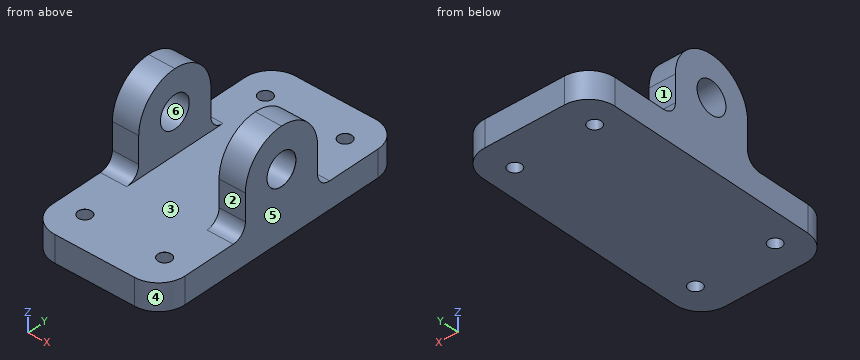
```python
from build123d import *

# Parameters (mm, degrees)
SKETCH1_W                        = 100
SKETCH1_H                        = 50
BOSS_EXTRUDE1_DEPTH              = 10
SKETCH2_W                        = 30
SKETCH2_H                        = 9.9
BOSS_EXTRUDE2_DEPTH              = 30
FILLET1_R                        = 15
F_12_0MM_DOWEL_HOLE1_D           = 12
F_12_0MM_DOWEL_HOLE1_CSINK_D     = 12.05
F_12_0MM_DOWEL_HOLE1_CSINK_ANGLE = 90
F_5_0MM_DOWEL_HOLE1_D            = 5
F_5_0MM_DOWEL_HOLE1_CSINK_D      = 5.05
F_5_0MM_DOWEL_HOLE1_CSINK_ANGLE  = 90
FILLET2_R                        = 5
FILLET3_R                        = 10


with BuildPart() as part:
    # Sketch1 → Boss-Extrude1 (new body)
    with BuildSketch(Plane(origin=(0, 0, 0), x_dir=(0, 1, 0), z_dir=(0, 0, 1))):
        Rectangle(SKETCH1_W, SKETCH1_H)
    extrude(amount=-BOSS_EXTRUDE1_DEPTH)

    # Sketch2 → Boss-Extrude2 (add)
    with BuildSketch(Plane(origin=(0, 0, 0), x_dir=(0, 1, 0), z_dir=(0, 0, 1))):
        with Locations((0, 20.05)):
            Rectangle(SKETCH2_W, SKETCH2_H)
        with Locations((0, -20.05)):
            Rectangle(SKETCH2_W, SKETCH2_H)
    extrude(amount=BOSS_EXTRUDE2_DEPTH)

    # Fillet1
    fillet1_edges = [part.edges().sort_by_distance(p)[0] for p in [
        (20.05, 15, 30),
        (20.05, -15, 30),
        (-20.05, 15, 30),
        (-20.05, -15, 30),
    ]]
    fillet(fillet1_edges, radius=FILLET1_R - 0.0001)  # a hair under: the kernel refuses the full size

    # Ø12.0mm Dowel Hole1 (through all)
    with Locations(Plane.YZ.offset(25)):
        with Locations((0, 15)):
            CounterSinkHole(F_12_0MM_DOWEL_HOLE1_D / 2, F_12_0MM_DOWEL_HOLE1_CSINK_D / 2, counter_sink_angle=F_12_0MM_DOWEL_HOLE1_CSINK_ANGLE)

    # Ø5.0mm Dowel Hole1 (through all)
    with Locations(Plane(origin=(0, 0, 0), x_dir=(0, 1, 0), z_dir=(0, 0, 1))):
        with Locations((37.5, -15), (-37.5, 15), (-37.5, -15), (37.5, 15)):
            CounterSinkHole(F_5_0MM_DOWEL_HOLE1_D / 2, F_5_0MM_DOWEL_HOLE1_CSINK_D / 2, counter_sink_angle=F_5_0MM_DOWEL_HOLE1_CSINK_ANGLE)

    # Fillet2
    fillet2_edges = [part.edges().sort_by_distance(p)[0] for p in [
        (-20.05, -15, 0),
        (-20.05, 15, 0),
        (20.05, -15, 0),
        (20.05, 15, 0),
    ]]
    fillet(fillet2_edges, radius=FILLET2_R)

    # Fillet3
    fillet3_edges = [part.edges().sort_by_distance(p)[0] for p in [
        (-25, -50, -5),
        (-25, 50, -5),
        (25, 50, -5),
        (25, -50, -5),
    ]]
    fillet(fillet3_edges, radius=FILLET3_R)


solid = part.part
```
Verification items for the finished model (mm, model axes). Face numbers are marked on the shaded views. A direction names the side the tool comes from. Round coordinates to 2 decimals unless told otherwise and drop trailing zeros. Write each loop counter-clockwise with the first axis right and the second up, starting at its lowest first coordinate (ties: lowest second). Pieces come first, ordered by that corner, then holes. Notation, with made-up numbers: (44, 79.5) - (81, 79.5) arc R23 cw to (81, 97.5) - close; hole circle Ø11 at (48, 24.25). An arc over 180 degrees is marked (long way). Answer as a JSON object with one key per item and string values. Group by question number.
Q1. Mould release check, pull along Y, two halves, no side actions. Record for the marked faces 4, 5 and 6: released by +Y, released by -Y, zero draft, split by the parting line, or undercut.
Q2. Thickness scan on line 1 (X direction, y = -8, z = 1.5); line 2 (X direction, y = 37.5, z = -5); line 3 (Z direction, x = -2, y = 16). Record the ranges inside material, lowest first.
Q3. Go/stop test with flat-tipped pins: pin 1 Ø5 at (x, z) = (-21.5, 11) entering from +Y; pin 2 Ø6.5 at (x, y) = (-15, 37.5) entering from +Z; pin 3 Ø9 at (y, z) = (-2, 14) entering from -X; pin 4 Ø5 at (x, z) = (-14, 7.5) entering from -Y. Record where each tip stops, or that it passes through.
Q4. Tool access check on the marked faces 1, 2 and 3. Record the directions out of +Z, -Z, +X, -X, +Y, -Y that give a thin tool (end or side, any length) a straight path to the whole face; none if there is none.
Q5. Section check C-C, the plane z = 12. Give the number of separate pieces and of enclosed holes in the cut face, plus the area to 3 significant figures.
Q6. Section check A-A, the plane y = -37.5. Enter the section's corners in (x, z) (3 decimals).
Q7. Section check D-D, the plane x = -6.5. Enter the section's corners in (y, z).
Found:
{
 "1": {"face 4": "released by -Y", "face 5": "zero draft", "face 6": "undercut"},
 "2": {"line 1": "x = -25 to -15.1, 15.1 to 25", "line 2": "x = -25 to -17.5, -12.5 to 12.5, 17.5 to 25", "line 3": "z = -10 to 0"},
 "3": {"pin 1": "stops at y = 15", "pin 2": "stops at z = 0", "pin 3": "stops at x = -25", "pin 4": "stops at y = -15"},
 "4": {"face 1": "+Z, +X, -X, +Y", "face 2": "+Z, +X, -X, -Y", "face 3": "+Z"},
 "5": {"separate pieces": "4", "enclosed holes": "0", "area": "388 mm^2"},
 "6": {"outline": "(-25, -10) - (-17.5, -10) - (-17.5, -0.025) - (-17.525, 0) - (-25, 0) - close; (-12.5, -10) - (12.5, -10) - (12.5, -0.025) - (12.475, 0) - (-12.475, 0) - (-12.5, -0.025) - close; (17.5, -10) - (25, -10) - (25, 0) - (17.525, 0) - (17.5, -0.025) - close"},
 "7": {"outline": "(-50, -10) - (50, -10) - (50, 0) - (-50, 0) - close"}
}
